Geometry check sheet. Reference: the model listing, model coordinates, mm. Face numbers are marked on the shaded views. Round coordinates to 2 decimals unless told otherwise and drop trailing zeros. Loops run counter-clockwise (first coordinate to the right, second up) from the corner with the lowest first, then second, coordinate; pieces in that order, holes last. Notation, with made-up numbers: (74.25, -24.75) - (79.25, -24.75) arc R21 ccw to (79.25, 3.25) - close; hole circle Ø10 at (72, 18). An arc over 180 degrees is marked (long way). Answer as CSV lines item,"result". Start each with the question number.
1) Cross-section at B-B on y = 53. Record the boundary of the cut face in (x, z), and give its area (3 significant figures).
2) Thickness scan on line 1 along X through (y, z) = (66, 16); line 2 along Y through (x, z) = (-41, 12); line 3 along Y through (x, z) = (48.4, 39.1). Record the ranges inside material, lowest first.
3) Depth check by flat-ended pin: P1, Ø0.6, axis at x = -53, z = 26, coming from the +Y side; P2, Ø5, axis at x = 27, y = -87, coming from the +Z side; P3, Ø1.6, axis at x = -53, z = 24.5, coming from the +Y side. Enter the tip coordinate at first touch or a pass-through.
4) Cross-section at A-A on z = 39. Record the boundary of the cut face in (x, y).
5) Draft check along X on the marked faces 1, 2, 3 and 4. Enter one of: released by +X, released by -X, zero draft, split by the parting line, or undercut.
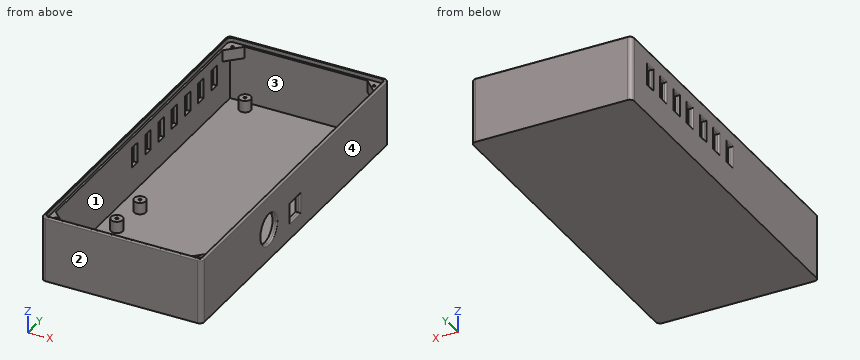
from build123d import *

# Parameters (mm, degrees)
F0_W      = 110
F0_H      = 240
F1_DEPTH  = 45
F2_W      = 104
F2_H      = 234
F3_DEPTH  = 42
F4_W      = 106.8
F4_H      = 236.8
F4_W_2    = 104
F4_H_2    = 234
F5_DEPTH  = 3
F6_R      = 4
F6_R_2    = 1
F7_DEPTH  = 8
F8_W      = 13
F8_H      = 13
F9_DEPTH  = 3
F10_W     = 7
F10_H     = 14
F11_DEPTH = 3
F12_R     = 3
F13_R     = 3
F15_DEPTH = 8
F17_DEPTH = 3
F18_D     = 2
F18_DEPTH = 6
F18_TIP   = 0.600860619
F19_R     = 1


# Not quite as in the source:
# - a feature names something its author has since deleted; it is built from what else it names


with BuildPart() as f1:
    # F0 (on Top) → F1 (new body)
    with BuildSketch(Plane.XY):
        Rectangle(F0_W, F0_H)
    extrude(amount=F1_DEPTH)

    # F2 (on face) → F3 (cut, through all)
    with BuildSketch(Plane.XY.offset(45)):
        Rectangle(F2_W, F2_H)
    extrude(amount=-F3_DEPTH, mode=Mode.SUBTRACT)

    # F4 (on face) → F5 (cut)
    with BuildSketch(Plane.XY.offset(45)):
        Rectangle(F4_W, F4_H)
        Rectangle(F4_W_2, F4_H_2, mode=Mode.SUBTRACT)
    extrude(amount=-F5_DEPTH, mode=Mode.SUBTRACT)

    # F6 (on face) → F7 (join)
    with BuildSketch(Plane.XY.offset(3)):
        with Locations((-38, 110)):
            Circle(F6_R)
        with Locations((-38, 110)):
            Circle(F6_R_2, mode=Mode.SUBTRACT)
        with Locations((38, 110)):
            Circle(F6_R)
        with Locations((38, 110)):
            Circle(F6_R_2, mode=Mode.SUBTRACT)
        with Locations((-38, -25)):
            Circle(F6_R)
        with Locations((-38, -25)):
            Circle(F6_R_2, mode=Mode.SUBTRACT)
        with Locations((38, -25)):
            Circle(F6_R)
        with Locations((38, -25)):
            Circle(F6_R_2, mode=Mode.SUBTRACT)
        with Locations((-40, -51)):
            Circle(F6_R)
        with Locations((-40, -51)):
            Circle(F6_R_2, mode=Mode.SUBTRACT)
        with Locations((40, -51)):
            Circle(F6_R)
        with Locations((40, -51)):
            Circle(F6_R_2, mode=Mode.SUBTRACT)
        with Locations((-40, -109)):
            Circle(F6_R)
        with Locations((-40, -109)):
            Circle(F6_R_2, mode=Mode.SUBTRACT)
        with Locations((40, -109)):
            Circle(F6_R)
        with Locations((40, -109)):
            Circle(F6_R_2, mode=Mode.SUBTRACT)
    extrude(amount=F7_DEPTH)

    # F8 (on face) → F9 (cut, through all)
    with BuildSketch(Plane.YZ.offset(55)):
        with Locations((-0.5, 18)):
            Rectangle(F8_W, F8_H)
    extrude(amount=-F9_DEPTH, mode=Mode.SUBTRACT)

    # F10 (on face) → F11 (cut, through all)
    with BuildSketch(Plane(origin=(-55, 0, 0), x_dir=(0, -1, 0), z_dir=(-1, 0, 0))):
        with Locations((-62.5, 28)):
            Rectangle(F10_W, F10_H)
        with Locations((-45.5, 28)):
            Rectangle(F10_W, F10_H)
        with Locations((-28.5, 28)):
            Rectangle(F10_W, F10_H)
        with Locations((-11.5, 28)):
            Rectangle(F10_W, F10_H)
        with Locations((5.5, 28)):
            Rectangle(F10_W, F10_H)
        with Locations((-79.5, 28)):
            Rectangle(F10_W, F10_H)
        with Locations((-96.5, 28)):
            Rectangle(F10_W, F10_H)
    extrude(amount=-F11_DEPTH, mode=Mode.SUBTRACT)

    # F12
    f12_edges = [f1.edges().sort_by_distance(p)[0] for p in [
        (-55, -120, 22.5),
        (55, -120, 22.5),
        (-55, 120, 22.5),
        (55, 120, 22.5),
    ]]
    fillet(f12_edges, radius=F12_R)

    # F13
    f13_edges = [f1.edges().sort_by_distance(p)[0] for p in [
        (-53.4, 118.4, 43.5),
        (53.4, 118.4, 43.5),
        (53.4, -118.4, 43.5),
        (-53.4, -118.4, 43.5),
    ]]
    fillet(f13_edges, radius=F13_R)

    # F14 (on face) → F15 (join)
    with BuildSketch(Plane.XY.offset(42)):
        Polygon((-42, 117), (-52, 117), (-52, 107), align=None)
        Polygon((52, 107), (52, 117), (42, 117), align=None)
        Polygon((42, -117), (52, -117), (52, -107), align=None)
        Polygon((-52, -107), (-52, -117), (-42, -117), align=None)
    extrude(amount=-F15_DEPTH)

    # F16 (on face) → F17 (cut, through all)
    with BuildSketch(Plane.YZ.offset(55)):
        with BuildLine():
            ThreePointArc((-33.9475087821, 11), (-26.699664275, 14.0021554928), (-23.6975087821, 21.25))
            ThreePointArc((-23.6975087821, 21.25), (-41.1953532893, 28.4978445072), (-33.9475087821, 11))
        make_face()
    extrude(amount=-F17_DEPTH, mode=Mode.SUBTRACT)

    # F18
    with Locations(Plane.XY.offset(42)):
        with Locations((48.4, 113.4), (-48.4, 113.4), (-48.4, -113.4), (48.4, -113.4)):
            Hole(F18_D / 2, depth=F18_DEPTH)
            with Locations((0, 0, -(F18_DEPTH + F18_TIP / 2))):  # 118° drill point
                Cone(0, F18_D / 2, F18_TIP, mode=Mode.SUBTRACT)

    # F19
    f19_edges = [f1.edges().sort_by_distance(p)[0] for p in [
        (0, -120, 45),
        (55, -33.947509, 31.5),
        (55, -7, 18),
        (55, -0.5, 11.5),
        (55, 6, 18),
        (55, -0.5, 24.5),
        (-55, 100, 28),
        (-55, 93, 28),
        (-55, 96.5, 21),
        (-55, 96.5, 35),
        (-55, 79.5, 35),
        (-55, 83, 28),
        (-55, 79.5, 21),
        (-55, 76, 28),
        (-55, 62.5, 35),
        (-55, 66, 28),
        (-55, 62.5, 21),
        (-55, 59, 28),
        (-55, 45.5, 35),
        (-55, 42, 28),
        (-55, 49, 28),
        (-55, 45.5, 21),
        (-55, 32, 28),
        (-55, 28.5, 21),
        (-55, 28.5, 35),
        (-55, 25, 28),
        (-55, 15, 28),
        (-55, 11.5, 21),
        (-55, 11.5, 35),
        (-55, 8, 28),
        (-55, -5.5, 35),
        (-55, -2, 28),
        (-55, -9, 28),
        (-55, -5.5, 21),
    ]]
    fillet(f19_edges, radius=F19_R)


solid = f1.part
Answer block:
1,outline,"(-55, 0) - (55, 0) - (55, 44) arc R1 ccw to (54, 45) - (53.4, 45) - (53.4, 42) - (52, 42) - (52, 3) - (-52, 3) - (-52, 42) - (-53.4, 42) - (-53.4, 45) - (-54, 45) arc R1 ccw to (-55, 44) - close"
1,area,"573 mm^2"
2,line 1,"x = -55 to -52, 52 to 55"
2,line 2,"y = -120 to -117, 117 to 120"
2,line 3,"y = -120 to -114.4, -112.4 to -110.6, 110.6 to 112.4, 114.4 to 120"
3,P1,"stops at y = 119.92"
3,P2,"stops at z = 3"
3,P3,"stops at y = 119.99"
4,outline,"(-55, -117) arc R3 ccw to (-52, -120) - (52, -120) arc R3 ccw to (55, -117) - (55, 117) arc R3 ccw to (52, 120) - (-52, 120) arc R3 ccw to (-55, 117) - close; hole (-52, -107) - (-42, -117) - (42, -117) - (52, -107) - (52, 107) - (42, 117) - (-42, 117) - (-52, 107) - close; hole circle Ø2 at (-48.4, -113.4); hole circle Ø2 at (-48.4, 113.4); hole circle Ø2 at (48.4, -113.4); hole circle Ø2 at (48.4, 113.4)"
5,face 1,"undercut"
5,face 2,"zero draft"
5,face 3,"undercut"
5,face 4,"released by +X"
